Read the model definition and answer for the solid it produces. Units are mm, in the model's axes. Face numbers are marked on the shaded views. A direction names the side the tool comes from. Give positions to 0.01 mm unless a question says otherwise; leave off trailing zeros. Order: outer loops, then holes, each group sorted by start corner. A loop starts at its lowest first (then second) coordinate and runs counter-clockwise, first axis right, second up. Notation, with made-up numbers: (54, -6) - (96, -6) arc R31 cw to (96, 33) - close; hole circle Ø7 at (-8, 8). An arc over 180 degrees is marked (long way). Use a Markdown table: item, result. Add a question column.
1. Consider L1, parallel to X at y = 312, z = 164; L2, parallel to Z at x = 317, y = 171.5; L3, parallel to Z at x = 202, y = 245.5. Determine where each line is inside the solid, lowest interval first.
2. Which of the six approach directions +Z, -Z, +X, -X, +Y, -Y give full straight-line access (tool end or side, diameter ignored) to the marked faces 1 and 2?
3. A cutting plane is placed at B-B on y = 58. Determine the outline of the cut face in (x, z).
4. For a pull along Y with two mould halves and no side action, classify the marked faces 3, 4 and 5 as released by +Y, released by -Y, zero draft, split by the parting line, or undercut.
5. Flat-ended cylindrical pins translate along their axes: P1, Ø12, axis at x = 261.5, z = 77, coming from the +Y side; P2, Ø6, axis at x = 104.5, y = 51.5, coming from the +Z side; P3, Ø6, axis at x = 290, y = 192, coming from the +Z side. Find the tip coordinate at first contact, or state that the pin passes through.
6. A cutting plane is placed at C-C on z = 21. Determine the outline of the cut face in (x, y), and give its area (3 significant figures).
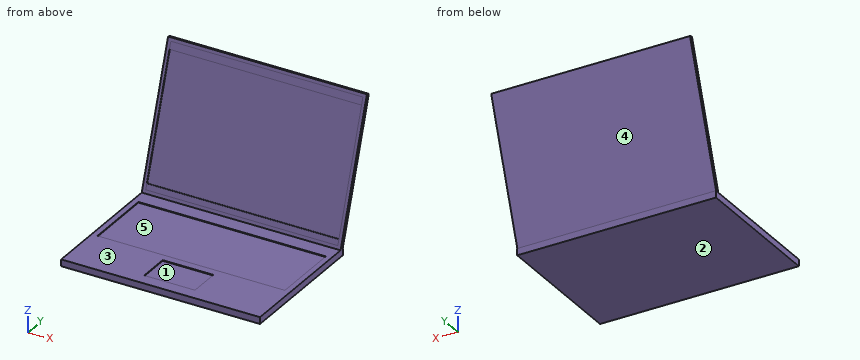
```python
from build123d import *

# Parameters (mm, degrees)
F1_DEPTH = 374.65
F2_W     = 361.95
F2_H     = 250.825
F3_DEPTH = 1.27
F4_W     = 353.1723869964
F4_H     = 130.2746757865
F4_W_2   = 95.635175705
F4_H_2   = 58.7365608662
F5_DEPTH = 1.27
F6_W     = 361.95
F6_H     = 13.6301602835
F6_H_2   = 10.7992181372
F7_DEPTH = 1.27


with BuildPart() as f1:
    # F0 (on Right) → F1 (new body)
    with BuildSketch(Plane.YZ):
        Polygon((256.4296126366, 0), (0, 0), (0, -12.7), (263.525, -12.7), (263.525, 0), (263.1285922031, 0), align=None)
        Polygon((340.3758903778, 249.7968135873), (256.4296126366, 0), (263.1285922031, 0), (346.3950907053, 247.774011714), align=None)
    extrude(amount=F1_DEPTH)

    # F2 (on face) → F3 (cut)
    with BuildSketch(Plane(origin=(0, 230.4084066856, -77.4306438252), x_dir=(1, 0, 0), z_dir=(0, -0.9479055634, 0.3185514761))):
        with Locations((187.325, 213.4485316231)):
            Rectangle(F2_W, F2_H)
    extrude(amount=-F3_DEPTH, mode=Mode.SUBTRACT)

    # F4 (on face) → F5 (cut)
    with BuildSketch(Plane.XY):
        with Locations((187.7015107311, 161.9020588696)):
            Rectangle(F4_W, F4_H)
        with Locations((190.7136440277, 52.3357847705)):
            Rectangle(F4_W_2, F4_H_2)
    extrude(amount=-F5_DEPTH, mode=Mode.SUBTRACT)

    # F6 (on face) → F7 (join, through all)
    with BuildSketch(Plane(origin=(0, 231.6122467511, -77.8352041999), x_dir=(1, 0, 0), z_dir=(0, -0.9479055634, 0.3185514761))):
        with Locations((187.325, 332.0459514814)):
            Rectangle(F6_W, F6_H)
        with Locations((187.325, 93.4356406917)):
            Rectangle(F6_W, F6_H_2)
    extrude(amount=F7_DEPTH)


solid = f1.part
```
Output values:
| question | item | result |
|---|---|---|
| 1 | L1 | 0 to 6.35, 368.3 to 374.65 |
| 1 | L2 | -12.7 to -1.27 |
| 1 | L3 | -12.7 to 0 |
| 2 | face 1 | +Z |
| 2 | face 2 | -Z, +X, -X, +Y, -Y |
| 3 | outline | (0, -12.7) - (374.65, -12.7) - (374.65, 0) - (238.53, 0) - (238.53, -1.27) - (142.9, -1.27) - (142.9, 0) - (0, 0) - close |
| 4 | face 3 | zero draft |
| 4 | face 4 | released by +Y |
| 4 | face 5 | undercut |
| 5 | P1 | y = 291.02 |
| 5 | P2 | z = 0 |
| 5 | P3 | z = -1.27 |
| 6 | outline | (0, 263.49) - (6.35, 263.49) - (6.35, 264.83) - (368.3, 264.83) - (368.3, 263.49) - (374.65, 263.49) - (374.65, 270.19) - (0, 270.19) - close |
| 6 | area | 2,020 mm² |
